```python
from build123d import *

# Parameters (mm, degrees)
SKETCH1_R           = 1.5
SKETCH1_R_2         = 2
BOSS_EXTRUDE1_DEPTH = 2


with BuildPart() as part:
    # Sketch1 → Boss-Extrude1 (new, symmetric)
    with BuildSketch(Plane(origin=(0, 0, 0), x_dir=(1, 0, 0), z_dir=(0, 1, 0))):
        with BuildLine():
            Line((-45.5, 32.5), (-45.5, -26.8))
            Line((-45.5, -26.8), (-55.5, -26.8))
            ThreePointArc((-55.5, -26.8), (-58.35, -29.65), (-55.5, -32.5))
            Line((-55.5, -32.5), (-45.5, -32.5))
            Line((-45.5, -32.5), (45.5, -32.5))
            Line((45.5, -32.5), (55.5, -32.5))
            ThreePointArc((55.5, -32.5), (58.35, -29.65), (55.5, -26.8))
            Line((55.5, -26.8), (45.5, -26.8))
            Line((45.5, -26.8), (45.5, 32.5))
            Line((45.5, 32.5), (45.5, 42.5))
            ThreePointArc((45.5, 42.5), (42.25, 45.75), (39, 42.5))
            Line((39, 42.5), (39, 32.5))
            Line((39, 32.5), (-39, 32.5))
            Line((-39, 32.5), (-39, 42.5))
            ThreePointArc((-39, 42.5), (-42.25, 45.75), (-45.5, 42.5))
            Line((-45.5, 42.5), (-45.5, 32.5))
        make_face()
        with Locations(Location((-42.25, 29.65, 0), (0, 0, 270))):
            Circle(SKETCH1_R, mode=Mode.SUBTRACT)
        with Locations(Location((42.25, 29.65, 0), (0, 0, 270))):
            Circle(SKETCH1_R, mode=Mode.SUBTRACT)
        with Locations(Location((42.25, -29.65, 0), (0, 0, 270))):
            Circle(SKETCH1_R, mode=Mode.SUBTRACT)
        with Locations(Location((-42.25, -29.65, 0), (0, 0, 270))):
            Circle(SKETCH1_R, mode=Mode.SUBTRACT)
        with Locations(Location((-42.25, 42.5, 0), (0, 0, 270))):
            Circle(SKETCH1_R_2, mode=Mode.SUBTRACT)
        with Locations(Location((42.25, 42.5, 0), (0, 0, 270))):
            Circle(SKETCH1_R_2, mode=Mode.SUBTRACT)
        with Locations(Location((-55.5, -29.65, 0), (0, 0, 270))):
            Circle(SKETCH1_R_2, mode=Mode.SUBTRACT)
        with Locations(Location((55.5, -29.65, 0), (0, 0, 270))):
            Circle(SKETCH1_R_2, mode=Mode.SUBTRACT)
    extrude(amount=BOSS_EXTRUDE1_DEPTH, both=True)


solid = part.part
```
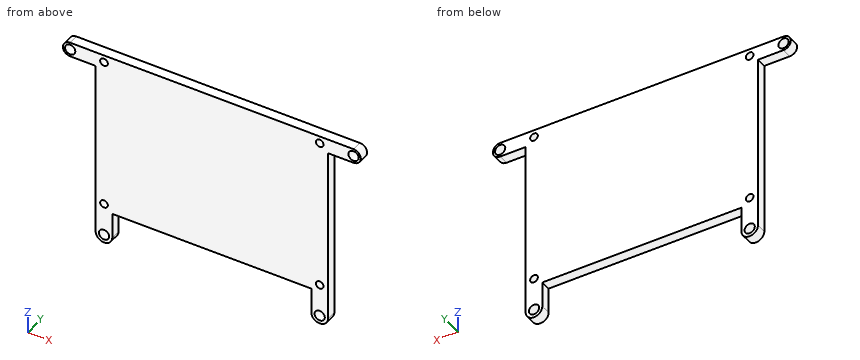
Can you work these out from the model? Positions are in its coordinate system, mm. Give positions to 0.01 mm unless a question says otherwise; leave off trailing zeros. Loops run counter-clockwise (first coordinate to the right, second up) from the corner with the lowest first, then second, coordinate; pieces in that order, holes last. Notation, with made-up numbers: M -22,13.5 L 22,13.5 A23 cw 22,34.5 Z; hole C -40,32.25 d10. An arc over 180 degrees is marked long. One line per question, with ' | ' between items. Start each with the question number.
Q1. If we section it at D-D (z = 29.65): Please give me the cut outline in (x, y), plus the area to 3 significant figures.
Q2. If I drill on line 1 (X direction, y = 0.8, z = 29.65); line 2 (X direction, y = 0.7, z = -42.5); line 3 (X direction, y = -1.2, z = -38), over which ranges is the centre line in solid material (lowest first)? Write a range as from..to.
Q3. If we section it at C-C (y = 0.55): State how many separate pieces and enclosed holes the cut face has, plus the area to 3 significant figures.
Q4. For pin 1 Ø3 at (x, z) = (-55.5, 29.65) entering from -Y; pin 2 Ø1.5 at (y, z) = (1.5, 18.5) entering from +X; pin 3 Ø2 at (x, y) = (-52.5, 0.5) entering from -Z; pin 4 Ø4.5 at (x, z) = (42.25, -42.5) entering from -Y, each with a flat end and sliding along its axis, tell me the tip position at first contact or that it passes through.
Q5. If we section it at A-A (x = -42.25): Please give me the cut outline in (y, z).
Q6. If we section it at B-B (z = -36): Please give me the cut outline in (x, y).
Computed:
1) outline: M -58.35,-2 L -57.5,-2 L -57.5,2 L -58.35,2 Z; M -53.5,-2 L -43.75,-2 L -43.75,2 L -53.5,2 Z; M -40.75,-2 L 40.75,-2 L 40.75,2 L -40.75,2 Z; M 43.75,-2 L 53.5,-2 L 53.5,2 L 43.75,2 Z; M 57.5,-2 L 58.35,-2 L 58.35,2 L 57.5,2 Z | area: 411 mm²
2) line 1: x = -58.35..-57.5, -53.5..-43.75, -40.75..40.75, 43.75..53.5, 57.5..58.35 | line 2: x = -45.5..-44.25, -40.25..-39, 39..40.25, 44.25..45.5 | line 3: x = -45.5..-39, 39..45.5
3) separate pieces: 1 | enclosed holes: 8 | area: 6,140 mm²
4) pin 1: passes through | pin 2: stops at x = 45.5 | pin 3: stops at z = 26.8 | pin 4: stops at y = -2
5) outline: M -2,-45.75 L 2,-45.75 L 2,-44.5 L -2,-44.5 Z; M -2,-40.5 L 2,-40.5 L 2,-31.15 L -2,-31.15 Z; M -2,-28.15 L 2,-28.15 L 2,28.15 L -2,28.15 Z; M -2,31.15 L 2,31.15 L 2,32.5 L -2,32.5 Z
6) outline: M -45.5,-2 L -39,-2 L -39,2 L -45.5,2 Z; M 39,-2 L 45.5,-2 L 45.5,2 L 39,2 Z
